Could you check a few things on this model? Use its own coordinates, in mm. A direction names the side the tool comes from. Give positions to 0.01 mm unless a question says otherwise; leave off trailing zeros. Loops run counter-clockwise (first coordinate to the right, second up) from the corner with the lowest first, then second, coordinate; pieces in that order, holes last. Notation, with made-up numbers: (13.25, -32.5) - (38.25, -32.5) arc R19 cw to (38.25, -9.5) - close; hole circle Ø10 at (-10.5, 86.5). An arc over 180 degrees is marked (long way). Write each question's results on one line, items separated by ' | '. Start each with the question number.
(1) For pin 1 (1 mm diameter, centred on y = 2, z = -4, fed in from -X); pin 2 (5 mm diameter, centred on x = 1.5, z = -5, fed in from -Y); pin 3 (5 mm diameter, centred on x = 0.5, z = -4, fed in from +Y); pin 4 (1 mm diameter, centred on x = -2, y = 1, fed in from +Z), each with a flat end and sliding along its axis, tell me the tip position at first contact or that it passes through.
(2) I need wall thicknesses on line 1 (Y direction, x = 0, z = -3.5); line 2 (Z direction, x = -3.5, y = 3); line 3 (X direction, y = -1, z = 1.5). Which ranges of each line are inside material? Lowest first, please.
(3) Suppose I cut it at C-C (z = -6.5). Please give me the cut outline in (x, y).
(4) On a 3-axis mill with a long thin cutter (end or side, diameter ignored), from which of +Z, -Z, +X, -X, +Y, -Y can I reach the whole of each face in a straight line? I mean faces 1 (the face through (-2, 4, 0)), 2 (the face through (0, 3, -8)). Say none if no direction works.
(5) Suppose I cut it at A-A (x = 0). Please give me the cut outline in (y, z), and give its area (3 significant figures).
(6) If we mould it in two halves opening along X, with no side actions, what happens to faces 3 (the face through (0.867, -3.905, -3.904)), 4 (the face through (-0.54, -2.44, -2.93)), 5 (the face through (2, -2, 2))? For each: released by +X, released by -X, zero draft, split by the parting line, or undercut.
from build123d import *

# Parameters (mm, degrees)
F2_R     = 2.5
F3_DEPTH = 10.001
F4_SIZE  = 0.3


with BuildPart() as f1:
    # F0 (on Front) → F1 (revolve)
    with BuildSketch(Plane.XZ):
        Polygon((0, 0), (0, 2), (-5, 2), (-5, 0), (-4, 0), (-4, -8), (0, -8), align=None)
    revolve(axis=Axis((0, 0, 0.636387), (0, 0, -1)))

    # F2 (on face) → F3 (cut, through all)
    with BuildSketch(Plane.XY.offset(2)):
        Circle(F2_R)
    extrude(amount=-F3_DEPTH, mode=Mode.SUBTRACT)

    # F4
    f4_edges = [f1.edges().sort_by_distance(p)[0] for p in [
        (5, 0, 2),
        (5, 0, 0),
        (4, 0, -8),
    ]]
    chamfer(f4_edges, length=F4_SIZE)


solid = f1.part
Output values:
1) pin 1: x = -3.71 | pin 2: y = -4 | pin 3: y = 4 | pin 4: z = 2
2) line 1: -4 to -2.5, 2.5 to 4 | line 2: 0 to 2 | line 3: -4.9 to -2.29, 2.29 to 4.9
3) outline: circle Ø8 at (0, 0); hole circle Ø5 at (0, 0)
4) face 1: -Z | face 2: -Z, +X, -X, +Y, -Y
5) outline: (-5, 0.3) - (-4.7, 0) - (-4, 0) - (-4, -7.7) - (-3.7, -8) - (-2.5, -8) - (-2.5, 2) - (-4.7, 2) - (-5, 1.7) - close; (2.5, -8) - (3.7, -8) - (4, -7.7) - (4, 0) - (4.7, 0) - (5, 0.3) - (5, 1.7) - (4.7, 2) - (2.5, 2) - close | area: 33.7 mm2
6) face 3: split by the parting line | face 4: undercut | face 5: zero draft
